from build123d import *

# Parameters (mm, degrees)
EXTRUDE_1_DEPTH     = 4
SKETCH_1_W          = 10
SKETCH_1_H          = 10
EXTRUDE_2_DEPTH     = 50
SKETCH_6_W          = 10
SKETCH_6_H          = 10
EXTRUDE_4_DEPTH     = 10
SKETCH_7_W          = 2
SKETCH_7_H          = 10
SKETCH_7_W_2        = 4.928830328
SKETCH_7_W_3        = 5.69296793
SKETCH_7_W_4        = 34
CUT_EXTRUDE_3_DEPTH = 28
CUT_EXTRUDE_4_DEPTH = 51
SKETCH_9_R          = 7
SKETCH_9_R_2        = 6
EXTRUDE_5_DEPTH     = 4


with BuildPart() as part:
    # 草图2 → 凸台-拉伸1 (new body)
    with BuildSketch(Plane(origin=(0, 0, 0), x_dir=(1, 0, 0), z_dir=(0, 1, 0))):
        Polygon((-5, -22), (5, -22), (5, -12), (15, -5), (25, -5), (25, 5), (-25, 5), (-25, -5), (-15, -5), (-5, -12), align=None)
    extrude(amount=EXTRUDE_1_DEPTH)

    # 草图1 → 凸台-拉伸2 (add)
    with BuildSketch(Plane(origin=(0, 0, 0), x_dir=(1, 0, 0), z_dir=(0, 1, 0))):
        with Locations((-20, 0)):
            Rectangle(SKETCH_1_W, SKETCH_1_H)
        with Locations((20, 0)):
            Rectangle(SKETCH_1_W, SKETCH_1_H)
    extrude(amount=-EXTRUDE_2_DEPTH)

    # 草图6 → 凸台-拉伸4 (add)
    with BuildSketch(Plane.XZ):
        with Locations((0, 17)):
            Rectangle(SKETCH_6_W, SKETCH_6_H)
    extrude(amount=EXTRUDE_4_DEPTH)

    # 草图7 → 切除-拉伸3 (cut, through all)
    with BuildSketch(Plane(origin=(0, 0, -5), x_dir=(-1, 0, 0), z_dir=(0, 0, -1))):
        with Locations((-24, -45)):
            Rectangle(SKETCH_7_W, SKETCH_7_H)
        with Locations((24, -45)):
            Rectangle(SKETCH_7_W, SKETCH_7_H)
        with Locations((-5.464415164, -5)):
            Rectangle(SKETCH_7_W_2, SKETCH_7_H)
        with Locations((5.846483965, -5)):
            Rectangle(SKETCH_7_W_3, SKETCH_7_H)
        with Locations((0, -45)):
            Rectangle(SKETCH_7_W_4, SKETCH_7_H)
    extrude(amount=-CUT_EXTRUDE_3_DEPTH, mode=Mode.SUBTRACT)

    # 草图8 → 切除-拉伸4 (cut, through all)
    with BuildSketch(Plane(origin=(25, 0, 0), x_dir=(0, 0, -1), z_dir=(1, 0, 0))):
        with BuildLine():
            Line((-22, -5), (-22, -14.409566658))
            Line((-22, -14.409566658), (-12, -14.409566658))
            Line((-12, -14.409566658), (-12, -5))
            ThreePointArc((-12, -5), (-17, -10), (-22, -5))
        make_face()
        with BuildLine():
            Line((-5, -45), (-5, -53.480862615))
            Line((-5, -53.480862615), (5, -53.480862615))
            Line((5, -53.480862615), (5, -45))
            ThreePointArc((5, -45), (0, -50), (-5, -45))
        make_face()
    extrude(amount=-CUT_EXTRUDE_4_DEPTH, mode=Mode.SUBTRACT)

    # 草图9 → 凸台-拉伸5 (add)
    with BuildSketch(Plane(origin=(0, 4, 0), x_dir=(1, 0, 0), z_dir=(0, 1, 0))):
        with Locations((0, -3.6)):
            Circle(SKETCH_9_R)
        with Locations((0, -3.6)):
            Circle(SKETCH_9_R_2, mode=Mode.SUBTRACT)
    extrude(amount=EXTRUDE_5_DEPTH)


solid = part.part
Could you check a few things on this model? Use its own coordinates, in mm. A direction names the side the tool comes from. Give positions to 0.01 mm unless a question says otherwise; leave off trailing zeros. Order: outer loops, then holes, each group sorted by start corner. A loop starts at its lowest first (then second) coordinate and runs counter-clockwise, first axis right, second up. Notation, with made-up numbers: (45.5, -17) - (61.5, -17) arc R5 cw to (61.5, -12) - close; hole circle Ø11 at (88.5, -40). An arc over 180 degrees is marked (long way). One line per item, written item: value. Start each with the question number.
1. For P1, Ø3.5, axis at x = 1, z = 2, coming from the +Y side; P2, Ø11, axis at y = -6.5, z = 18, coming from the +X side; P3, Ø3, axis at y = -44, z = 0.5, coming from the +X side, each with a flat end and sliding along its axis, tell me the tip position at first contact or that it passes through.
2. If I drill on probe 1 along X at (y, z) = (6.1, 3.6); probe 2 along Z at (x, y) = (0, 5.9); probe 3 along Y at (x, z) = (-18.5, 0.25), over which ranges is the centre line in solid material (lowest first)?
3. Imagine slicing it at C-C on x = 0. List the corners of the cut face in (y, z) for me.
4. For faces 1 (the face through (24, -40, 0)), 2 (the face through (-4.42, 5.97, -0.46)), 3 (the face through (-3, -5, 17)), 4 (the face through (16, -40, 0)), 5 (the face through (0, -2, 12)), which set-ups out of +Z, -Z, +X, -X, +Y, -Y let a thin tool reach every point of the face, with its end or its side?
5. Imagine slicing it at B-B on z = 17. List the corners of the cut face in (x, y) for me.
6. Thinking about a two-plate mould opening in X: for faces 6 (the face through (25, -18, 0)), 7 (the face through (-6, 4, -1)), 8 (the face through (0, 0, 5)), which applies, +X half, -X half, draft (parallel to the pull), parting line (faces both ways), or undercut?
7. Imagine slicing it at D-D on y = -46. List the corners of the cut face in (x, z) for me.
8. Imagine slicing it at A-A on y = -30. List the corners of the cut face in (x, z) for me.
Values:
1. P1: y = 4
1. P2: x = 3
1. P3: x = 23
2. probe 1: -7 to -6, 6 to 7
2. probe 2: -3.4 to -2.4, 9.6 to 10.6
2. probe 3: -49.99 to 4
3. outline: (-5, 12) - (0, 12) - (0, -5) - (4, -5) - (4, -3.4) - (8, -3.4) - (8, -2.4) - (4, -2.4) - (4, 9.6) - (8, 9.6) - (8, 10.6) - (4, 10.6) - (4, 22) - (-5, 22) arc R5 ccw to start
4. face 1: +Z, -Z, +X, -Y
4. face 2: +Y
4. face 3: +Z, -Z, -X, -Y
4. face 4: +Z, -Z, -Y
4. face 5: -Z, +X, -X, -Y
5. outline: (-5, 0) - (-3, 0) - (-3, -10) - (3, -10) - (3, 0) - (5, 0) - (5, 4) - (-5, 4) - close
6. face 6: +X half
6. face 7: draft
6. face 8: undercut
7. outline: (-23, -4.9) - (-17, -4.9) - (-17, 4.9) - (-23, 4.9) - close; (17, -4.9) - (23, -4.9) - (23, 4.9) - (17, 4.9) - close
8. outline: (-25, -5) - (-15, -5) - (-15, 5) - (-25, 5) - close; (15, -5) - (25, -5) - (25, 5) - (15, 5) - close
